```python
from build123d import *

# Parameters (mm, degrees)
F1_DEPTH = 57.1754
F2_T     = -0.635
F3_ANGLE = 90


with BuildPart() as f1:
    # F0 (on Top) → F1 (new body)
    with BuildSketch(Plane.XY):
        with BuildLine():
            ThreePointArc((57.785, 25.9715), (54.046657, 34.996657), (45.0215, 38.735))
            Line((45.0215, 38.735), (-45.0215, 38.735))
            ThreePointArc((-45.0215, 38.735), (-54.046657, 34.996657), (-57.785, 25.9715))
            Line((-57.785, 25.9715), (-57.785, -25.9715))
            ThreePointArc((-57.785, -25.9715), (-54.046657, -34.996657), (-45.0215, -38.735))
            Line((-45.0215, -38.735), (45.0215, -38.735))
            ThreePointArc((45.0215, -38.735), (54.046657, -34.996657), (57.785, -25.9715))
            Line((57.785, -25.9715), (57.785, 25.9715))
        make_face()
    extrude(amount=F1_DEPTH)

    # F2
    f2_openings = [f1.faces().sort_by_distance(p)[0] for p in [
        (0, 0, 57.1754),
        (0, 0, 0),
    ]]
    offset(amount=F2_T, openings=f2_openings)


with BuildPart() as f1_1:
    # F3: moved
    add(f1.part.rotate(Axis((0, -38.735, 0), (-1, 0, 0)), F3_ANGLE))


solid = f1_1.part
```
Geometry check sheet. Reference: the model listing, model coordinates, mm. A direction names the side the tool comes from. Coordinates: 2 decimals unless noted, no trailing zeros. Order: outer loops, then holes, each group sorted by start corner. A loop starts at its lowest first (then second) coordinate and runs counter-clockwise, first axis right, second up. Notation, with made-up numbers: (-34.5, 0) - (-28.5, 0) arc R20 cw to (-28.5, 19) - close; hole circle Ø6 at (64.5, -10.5). An arc over 180 degrees is marked (long way). Answer in a Markdown table with one row per item. Add a question column.
1. Material ranges on L1, parallel to X at y = -6, z = -23.5 (3 decimals); L2, parallel to Z at x = 27, y = -34.5 (3 decimals); L3, parallel to X at y = -28, z = -12.5, recorded low to high. Write a range as [from, to].
2. Draft check along X on faces 1 (the face through (57.15, -11, -38)), 2 (the face through (54.145, -10.548, -73.632)), 3 (the face through (1, -11, -77.47)), 4 (the face through (-57.15, -11, -39)). Enter one of: +X half, -X half, draft (parallel to the pull), parting line (faces both ways), or undercut.
3. Section check A-A (x = -38.5). Enter the section's corners in (y, z) (3 decimals), plus the area to 3 significant figures.
4. Section check B-B (z = -39.5). Enter the section's corners in (x, y) (3 decimals), plus the area to 3 significant figures.
5. Gauge pin test, flat end, axial feed: pin 1 Ø1 at (y, z) = (8.5, -9) entering from +X. Record the tip position at first contact, or that the pin passes through.
6. Access from +Z, -Z, +X, -X, +Y, -Y to the whole of each face (thin tool, end or side, straight path). Record for faces 5 (the face through (-1, -11, 0)), 6 (the face through (-53.5, -10.55, -73.38)).
Data:
| question | item | result |
|---|---|---|
| 1 | L1 | x = [-57.785, -57.15], [57.15, 57.785] |
| 1 | L2 | z = [-77.47, -76.835], [-0.635, 0] |
| 1 | L3 | x = [-57.78, -57.15], [57.15, 57.78] |
| 2 | face 1 | undercut |
| 2 | face 2 | +X half |
| 2 | face 3 | draft |
| 2 | face 4 | undercut |
| 3 | outline | (-38.735, -77.47) - (18.44, -77.47) - (18.44, -76.835) - (-38.735, -76.835) - close; (-38.735, -0.635) - (18.44, -0.635) - (18.44, 0) - (-38.735, 0) - close |
| 3 | area | 72.6 mm² |
| 4 | outline | (-57.785, -38.735) - (-57.15, -38.735) - (-57.15, 18.44) - (-57.785, 18.44) - close; (57.15, -38.735) - (57.785, -38.735) - (57.785, 18.44) - (57.15, 18.44) - close |
| 4 | area | 72.6 mm² |
| 5 | pin 1 | stops at x = 57.36 |
| 6 | face 5 | +Z, +X, -X, +Y, -Y |
| 6 | face 6 | +Y, -Y |
